Input: part model. Units: mm. Frame: model coordinates. A direction names the side the tool comes from. Round coordinates to 2 decimals unless told otherwise and drop trailing zeros. Loops run counter-clockwise (first coordinate to the right, second up) from the corner with the lowest first, then second, coordinate; pieces in that order, holes last. Notation, with made-up numbers: (65.5, -12.75) -> (114.5, -12.75) arc R14 ccw to (114.5, 2.25) -> close; hole circle Ø10 at (63.25, 88.25). An arc over 180 degrees is marked (long way). Answer as a JSON object with one key per item and string values. Group by question number.
Item 1: Set-up query: faces 1 (the cylindrical face through (277.9, -30.22, 2.5)), 2 (the flat face through (235, -25.4, 2)). Return all of +Z, -Z, +X, -X, +Y, -Y with unobstructed straight access to the full face (end or side cutting, diameter ignored); none if empty.
Item 2: Material intervals for line 1 (Y direction, x = 269, z = 1.8); line 2 (X direction, y = -17, z = 2.15), sorted ascending. Write a range as [from, to].
Item 3: Draft query along Y for faces 3 (the flat face through (196.802, -16, 2)), 4 (the cylindrical face through (272.09, -24.45, 2.41)), 5 (the cylindrical face through (277.9, -1.53, 2.5)), 6 (the cylindrical face through (191.98, -30.3, 2.06)). Return one class per face: released by +Y, released by -Y, zero draft, split by the parting line, or undercut.
Item 4: Section query B-B on z = 2. Return loops of the section in (x, y) (3 decimals).
Item 5: Section query A-A on y = -14. Return loops of the section in (x, z).
Item 6: Section query D-D on y = -1.5. Return loops of the section in (x, z), and give its area (3 significant figures).
Item 7: Section query C-C on x = 251.5. Return loops of the section in (y, z), and give its area (3 significant figures).
from build123d import *

# Parameters (mm, degrees)
F4_DEPTH = 31.75
F6_DEPTH = 4.937656
F7_R     = 5.08


with BuildPart() as f4:
    # F3 (on face) → F4 (new body)
    with BuildSketch(Plane.XZ):
        Polygon((279.348608, 0), (279.348608, 4.936656), (190.452309, 4.125477), (190.452309, 0), align=None)
    extrude(amount=F4_DEPTH)

    # F5 (on face) → F6 (cut, through all)
    with BuildSketch(Plane(origin=(0, 0, 0), x_dir=(1, 0, 0), z_dir=(0, 0, -1))):
        with BuildLine():
            Line((269.823608, 25.4), (199.977309, 25.4))
            ThreePointArc((199.977309, 25.4), (197.732245, 24.470064), (196.802309, 22.225))
            Line((196.802309, 22.225), (196.802309, 9.525))
            ThreePointArc((196.802309, 9.525), (197.732245, 7.279936), (199.977309, 6.35))
            Line((199.977309, 6.35), (269.823608, 6.35))
            ThreePointArc((269.823608, 6.35), (272.068672, 7.279936), (272.998608, 9.525))
            Line((272.998608, 9.525), (272.998608, 22.225))
            ThreePointArc((272.998608, 22.225), (272.068672, 24.470064), (269.823608, 25.4))
        make_face()
    extrude(amount=-F6_DEPTH, mode=Mode.SUBTRACT)

    # F7
    f7_edges = [f4.edges().sort_by_distance(p)[0] for p in [
        (279.348608, -31.75, 2.468328),
        (190.452309, -31.75, 2.062739),
        (190.452309, 0, 2.062739),
        (279.348608, 0, 2.468328),
    ]]
    fillet(f7_edges, radius=F7_R)


solid = f4.part
Solved:
{
 "1": {"face 1": "+Z, -Z, +X, -Y", "face 2": "+Z, -Z"},
 "2": {"line 1": "[-31.75, -25.4], [-6.35, 0]", "line 2": "[190.45, 196.8], [273, 279.35]"},
 "3": {"face 3": "undercut", "face 4": "undercut", "face 5": "released by +Y", "face 6": "released by -Y"},
 "4": {"outline": "(190.452, -26.67) arc R5.08 ccw to (195.532, -31.75) -> (274.269, -31.75) arc R5.08 ccw to (279.349, -26.67) -> (279.349, -5.08) arc R5.08 ccw to (274.269, 0) -> (195.532, 0) arc R5.08 ccw to (190.452, -5.08) -> close; hole (196.802, -22.225) arc R3.175 ccw to (199.977, -25.4) -> (269.824, -25.4) arc R3.175 ccw to (272.999, -22.225) -> (272.999, -9.525) arc R3.175 ccw to (269.824, -6.35) -> (199.977, -6.35) arc R3.175 ccw to (196.802, -9.525) -> close"},
 "5": {"outline": "(190.45, 0) -> (196.8, 0) -> (196.8, 4.18) -> (190.45, 4.13) -> close; (273, 0) -> (279.35, 0) -> (279.35, 4.94) -> (273, 4.88) -> close"},
 "6": {"outline": "(191.93, 0) -> (277.87, 0) -> (277.87, 4.92) -> (191.93, 4.14) -> close", "area": "389 mm²"},
 "7": {"outline": "(-31.75, 0) -> (-25.4, 0) -> (-25.4, 4.68) -> (-31.75, 4.68) -> close; (-6.35, 0) -> (0, 0) -> (0, 4.68) -> (-6.35, 4.68) -> close", "area": "59.5 mm²"}
}
